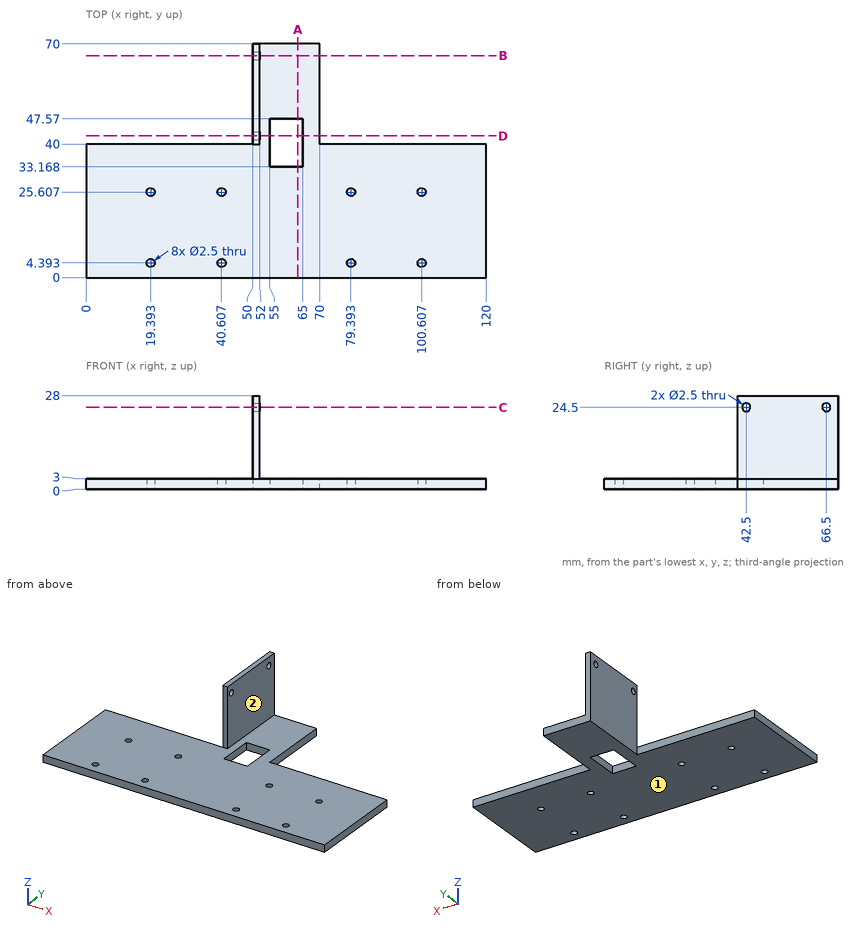
Geometry: see drawing. Coordinates: mm, zero at the bounding-box minimum. A direction names the side the tool comes from. Give positions to 0.01 mm unless a question says otherwise; leave off trailing zeros. Order: outer loops, then holes, each group sorted by start corner. A loop starts at its lowest first (then second) coordinate and runs counter-clockwise, first axis right, second up. Notation, with made-up numbers: (71, -30) -> (87, -30) arc R13 ccw to (87, -6) -> close; hole circle Ø8 at (60.5, 62). An arc over 180 degrees is marked (long way). Write each question's results on one line, items separated by ' | '.
1) Line query: line 1 along Y through (x, z) = (50.75, 24.5); line 2 along Z through (x, y) = (81, 27); line 3 along X through (y, z) = (63, 20). Output: solid intervals per line, ascending.
Geometry says:
line 1: y = 40 to 41.25, 43.75 to 65.25, 67.75 to 70 | line 2: z = 0 to 3 | line 3: x = 50 to 52
2) First-contact query: pin 1 Ø3 at (y, z) = (22, 4) entering from +X; pin 2 Ø1.6 at (x, z) = (51, 20) entering from -Y; pin 3 Ø3.5 at (x, z) = (91, 1.5) entering from +Y; pin 4 Ø2.5 at (y, z) = (42.5, 2) entering from -X. Flat tips, straight axial feed; report the tip coordinate or a pass-through.
Geometry says:
pin 1: stops at x = 120 | pin 2: stops at y = 40 | pin 3: stops at y = 40 | pin 4: stops at x = 50
3) Set-up query: the marked faces 1 and 2. Return all of +Z, -Z, +X, -X, +Y, -Y with unobstructed straight access to the full face (end or side cutting, diameter ignored); none if empty.
Geometry says:
face 1: -Z, +X, -X, +Y, -Y | face 2: +Z, +X, +Y, -Y
4) Cut plane B-B (y = 66.5). Output: boundary loops of the cut face in (x, z).
Geometry says:
outline: (50, 0) -> (70, 0) -> (70, 3) -> (52, 3) -> (52, 23.25) -> (50, 23.25) -> close; (50, 25.75) -> (52, 25.75) -> (52, 28) -> (50, 28) -> close
5) Cut plane C-C (z = 24.5). Output: boundary loops of the cut face in (x, y).
Geometry says:
outline: (50, 40) -> (52, 40) -> (52, 41.25) -> (50, 41.25) -> close; (50, 43.75) -> (52, 43.75) -> (52, 65.25) -> (50, 65.25) -> close; (50, 67.75) -> (52, 67.75) -> (52, 70) -> (50, 70) -> close
6) Cut plane D-D (y = 42.5). Output: boundary loops of the cut face in (x, z).
Geometry says:
outline: (50, 0) -> (55, 0) -> (55, 3) -> (52, 3) -> (52, 23.25) -> (50, 23.25) -> close; (50, 25.75) -> (52, 25.75) -> (52, 28) -> (50, 28) -> close; (65, 0) -> (70, 0) -> (70, 3) -> (65, 3) -> close
7) Cut plane A-A (x = 63.5). Output: boundary loops of the cut face in (y, z), and give its area (3 significant figures).
Geometry says:
outline: (0, 0) -> (33.17, 0) -> (33.17, 3) -> (0, 3) -> close; (47.57, 0) -> (70, 0) -> (70, 3) -> (47.57, 3) -> close | area: 167 mm²
